```python
from build123d import *

# Parameters (mm, degrees)
EXTRUDE_1_DEPTH     = 15
EXTRUDE_1_2_DEPTH   = 15
SKETCH_1_W          = 55
SKETCH_1_H          = 4
EXTRUDE_1_3_DEPTH   = 15
EXTRUDE_2_DEPTH     = 4
EXTRUDE_3_DEPTH     = 20
SKETCH_4_R          = 1.8
CUT_EXTRUDE_1_DEPTH = 20
SKETCH_5_R          = 1.8
CUT_EXTRUDE_2_DEPTH = 20


with BuildPart() as part:
    # Sketch 1 → Extrude 1 (new body)
    with BuildSketch(Plane(origin=(0, 0, 0), x_dir=(1, 0, 0), z_dir=(0, 1, 0))):
        Polygon((-24.755102041, 11.775510204), (-4.755102041, 11.775510204), (-4.755102041, 31.775510204), (-8.755102041, 31.775510204), (-8.755102041, 15.775510204), (-24.755102041, 15.775510204), align=None)
    extrude(amount=EXTRUDE_1_DEPTH)



with BuildPart() as body_2:
    # Sketch 1 → Extrude 1 2 (new body)
    with BuildSketch(Plane(origin=(0, 0, 0), x_dir=(1, 0, 0), z_dir=(0, 1, 0))):
        Polygon((30.244897959, 15.775510204), (14.244897959, 15.775510204), (14.244897959, 31.775510204), (10.244897959, 31.775510204), (10.244897959, 11.775510204), (12.244897959, 11.775510204), (30.244897959, 11.775510204), align=None)
    extrude(amount=EXTRUDE_1_2_DEPTH)


with BuildPart() as body_3:
    # Sketch 1 → Extrude 1 3 (new body)
    with BuildSketch(Plane(origin=(0, 0, 0), x_dir=(1, 0, 0), z_dir=(0, 1, 0))):
        with Locations((2.744897959, -5.224489796)):
            Rectangle(SKETCH_1_W, SKETCH_1_H)
    extrude(amount=EXTRUDE_1_3_DEPTH)


with BuildPart() as part_1:
    add(part.part)

    add(body_2.part)  # Extrude 2 merges body 2

    add(body_3.part)  # Extrude 2 merges body 3
    # Sketch 2 → Extrude 2 (add)
    with BuildSketch(Plane.XZ):
        Polygon((-8.755102041, -15.775510204), (-24.755102041, -15.775510204), (-24.755102041, 7.224489796), (30.244897959, 7.224489796), (30.244897959, -15.775510204), (14.244897959, -15.775510204), (14.244897959, -31.775510204), (-8.755102041, -31.775510204), align=None)
    extrude(amount=EXTRUDE_2_DEPTH)

    # Sketch 3 → Extrude 3 (add)
    with BuildSketch(Plane(origin=(0, 15, 0), x_dir=(1, 0, 0), z_dir=(0, 1, 0))):
        Polygon((-8.755102041, 15.775510204), (-4.755102041, 15.775510204), (-4.755102041, -3.224489796), (10.244897959, -3.224489796), (10.244897959, 11.675510204), (14.244897959, 11.675510204), (14.244897959, -7.224489796), (10.244897959, -7.224489796), (-4.755102041, -7.224489796), (-8.755102041, -7.224489796), align=None)
    extrude(amount=EXTRUDE_3_DEPTH)

    # Sketch 4 → Cut-Extrude 1 (cut)
    with BuildSketch(Plane.XZ.offset(4)):
        with Locations((2.744897959, -24.275510204)):
            Circle(SKETCH_4_R)
        with Locations((2.744897959, -4.275510204)):
            Circle(SKETCH_4_R)
    extrude(amount=-CUT_EXTRUDE_1_DEPTH, mode=Mode.SUBTRACT)

    # Sketch 5 → Cut-Extrude 2 (cut)
    with BuildSketch(Plane.XY.offset(7.224489796)):
        with Locations((2.744897959, 27.5)):
            Circle(SKETCH_5_R)
    extrude(amount=-CUT_EXTRUDE_2_DEPTH, mode=Mode.SUBTRACT)


solid = part_1.part
```
Could you check a few things on this model? Use its own coordinates, in mm. A direction names the side the tool comes from. Coordinates: 2 decimals unless noted, no trailing zeros. Loops run counter-clockwise (first coordinate to the right, second up) from the corner with the lowest first, then second, coordinate; pieces in that order, holes last. Notation, with made-up numbers: M -26,45 L 32,45 A31 cw 32,69 Z; hole C 14.5,-3.5 d2. An arc over 180 degrees is marked long. Put each result on its own line as item: value. Start each with the question number.
(1) Suppose I cut it at C-C on x = 20.5. Please give me the cut outline in (y, z).
(2) Suppose I cut it at B-B on z = -8.5. Please give me the cut outline in (x, y), then the cut area to 3 significant figures.
(3) I need wall thicknesses on line 1 (Z direction, x = -14, y = 13); line 2 (X direction, y = 6.5, z = -12); line 3 (X direction, y = 29, z = -11.5). Which ranges of each line are inside material? Lowest first, please. Write a range as from..to.
(4) Suppose I cut it at A-A on y = 3. Please give me the cut outline in (x, z), then the cut area to 3 significant figures.
(5) Thinking about a two-plate mould opening in Z: for faces 1 (the face through (22, 15, 5)), 2 (the face through (12, 15, -4)), 3 (the face through (22, 6, -15.776)), 4 (the face through (20, 7, -11.776)), which applies, pulls with the +Z half, pulls with the -Z half, needs draft (parallel to the pull), parting line crosses it, or undercut?
(6) Will these pins go through, and if not, where does the flat tip stop? P1, Ø10, axis at y = 0.5, z = -22, coming from the -X side; P2, Ø4.5, axis at x = 12.5, y = 24, coming from the -Z side; P3, Ø10, axis at x = 19, z = -20.5, coming from the +Y side; P4, Ø3, axis at x = 2.74, z = -24.28, coming from the -Y side.
(7) For faces 5 (the face through (-8.755, 6, -24)), 6 (the face through (-17, 15, -14)), 7 (the face through (-7, 15, -24)), 8 (the face through (-4.755, 17, -15)), 9 (the face through (13, 15, -17)), which set-ups out of +Z, -Z, +X, -X, +Y, -Y let a thin tool reach every point of the face, with its end or its side?
(8) Suppose I cut it at D-D on y = 27.5. Please give me the cut outline in (x, z), then the cut area to 3 significant figures.
Solutions:
1. outline: M -4,-15.78 L 15,-15.78 L 15,-11.78 L 0,-11.78 L 0,3.22 L 15,3.22 L 15,7.22 L -4,7.22 Z
2. outline: M -24.76,-4 L 30.24,-4 L 30.24,0 L -24.76,0 Z; M -8.76,15 L -4.76,15 L -4.76,35 L -8.76,35 Z; M 10.24,15 L 14.24,15 L 14.24,35 L 10.24,35 Z
2. area: 380 mm2
3. line 1: z = -15.78..-11.78, 3.22..7.22
3. line 2: x = -24.76..-4.76, 10.24..30.24
3. line 3: x = -8.76..-4.76, 10.24..14.24
4. outline: M -24.76,-15.78 L -8.76,-15.78 L -8.76,-31.78 L -4.76,-31.78 L -4.76,-11.78 L -24.76,-11.78 Z; M -24.76,3.22 L 30.24,3.22 L 30.24,7.22 L -24.76,7.22 Z; M 10.24,-31.78 L 14.24,-31.78 L 14.24,-15.78 L 30.24,-15.78 L 30.24,-11.78 L 10.24,-11.78 Z
4. area: 508 mm2
5. face 1: needs draft
5. face 2: undercut
5. face 3: pulls with the -Z half
5. face 4: undercut
6. P1: stops at x = -8.76
6. P2: stops at z = -11.68
6. P3: stops at y = 15
6. P4: passes through
7. face 5: -Z, -X, +Y, -Y
7. face 6: +Z, -Z, -X, +Y
7. face 7: -Z, +X, -X, +Y
7. face 8: -Z, +Y
7. face 9: -Z, +X, +Y
8. outline: M -8.76,-15.78 L -4.76,-15.78 L -4.76,3.22 L 0.94,3.22 L 0.94,7.22 L -8.76,7.22 Z; M 4.54,3.22 L 10.24,3.22 L 10.24,-11.68 L 14.24,-11.68 L 14.24,7.22 L 4.54,7.22 Z
8. area: 213 mm2
